Work out the finished part from the listing and answer in its coordinate system (mm). Round coordinates to 2 decimals unless told otherwise and drop trailing zeros. Loops run counter-clockwise (first coordinate to the right, second up) from the corner with the lowest first, then second, coordinate; pieces in that order, holes last. Notation, with made-up numbers: (11.5, 62.5) - (25.5, 62.5) arc R23 ccw to (25.5, 71.5) - close; hole circle Ø9 at (64.5, 83). An arc over 180 degrees is marked (long way). Use CSV: the item, a comma, the result in double quotes. Start each with the question number.
from build123d import *

# Parameters (mm, degrees)
ESQUISSE1_W                                 = 100
ESQUISSE1_H                                 = 100
BOSS_EXTRU_1_DEPTH                          = 1
FRAISAGE_POUR_VIS_T_TE_FRAIS_E_M31_AT_COUNT = 2
FRAISAGE_POUR_VIS_T_TE_FRAIS_E_M31_AT_PITCH = 90
FRAISAGE_POUR_VIS_T_TE_FRAIS_E_M31_2_COUNT  = 2
FRAISAGE_POUR_VIS_T_TE_FRAIS_E_M31_2_PITCH  = 127.279220614
FRAISAGE_POUR_VIS_T_TE_FRAIS_E_M31_3_COUNT  = 2
FRAISAGE_POUR_VIS_T_TE_FRAIS_E_M31_3_PITCH  = 90
ESQUISSE4_R                                 = 5.05
ESQUISSE4_R_2                               = 1
ENL_V_MAT_EXTRU_1_DEPTH                     = 2


with BuildPart() as part:
    # Esquisse1 → Boss.-Extru.1 (new body)
    with BuildSketch(Plane.XY):
        with Locations((50, 50)):
            Rectangle(ESQUISSE1_W, ESQUISSE1_H)
    extrude(amount=BOSS_EXTRU_1_DEPTH)

    # Esquisse3 → Fraisage pour vis à tête fraisée M31 (revolve, cut)
    with BuildSketch(Plane(origin=(5, 95, 1), x_dir=(0, -1, 0), z_dir=(1, 0, 0))):
        Polygon((0, 0), (0, 1), (1.8, 1), (1.8, 1.35), (3.15, 0), align=None)
    fraisage_pour_vis_t_te_frais_e_m31 = revolve(axis=Axis((5, 95, 7.35), (0, 0, -1)), mode=Mode.SUBTRACT)

    # Fraisage pour vis à tête fraisée M31 at: Fraisage pour vis à tête fraisée M31 ×2
    with Locations(*[(i * FRAISAGE_POUR_VIS_T_TE_FRAIS_E_M31_AT_PITCH, 0, 0) for i in range(1, FRAISAGE_POUR_VIS_T_TE_FRAIS_E_M31_AT_COUNT)]):
        add(fraisage_pour_vis_t_te_frais_e_m31, mode=Mode.SUBTRACT)

    # Fraisage pour vis _ t_te frais_e M31 2: Fraisage pour vis à tête fraisée M31 ×2
    with Locations(*[Vector(0.707106781, -0.707106781, 0) * (i * FRAISAGE_POUR_VIS_T_TE_FRAIS_E_M31_2_PITCH) for i in range(1, FRAISAGE_POUR_VIS_T_TE_FRAIS_E_M31_2_COUNT)]):
        add(fraisage_pour_vis_t_te_frais_e_m31, mode=Mode.SUBTRACT)

    # Fraisage pour vis _ t_te frais_e M31 3: Fraisage pour vis à tête fraisée M31 ×2
    with Locations(*[(0, -i * FRAISAGE_POUR_VIS_T_TE_FRAIS_E_M31_3_PITCH, 0) for i in range(1, FRAISAGE_POUR_VIS_T_TE_FRAIS_E_M31_3_COUNT)]):
        add(fraisage_pour_vis_t_te_frais_e_m31, mode=Mode.SUBTRACT)

    # Esquisse4 → Enlèv. mat.-Extru.1 (cut, through all)
    with BuildSketch(Plane.XY.offset(1)):
        with Locations((12.5, 75)):
            Circle(ESQUISSE4_R)
        with Locations((12.5, 25)):
            Circle(ESQUISSE4_R_2)
        with Locations((10, 19.5)):
            Circle(ESQUISSE4_R_2)
        with Locations((7, 25)):
            Circle(ESQUISSE4_R_2)
        with Locations((18, 25)):
            Circle(ESQUISSE4_R_2)
        with Locations((10, 30.5)):
            Circle(ESQUISSE4_R_2)
        with Locations((15, 30.5)):
            Circle(ESQUISSE4_R_2)
        with Locations((15, 19.5)):
            Circle(ESQUISSE4_R_2)
        with Locations((12.5, 60)):
            Circle(ESQUISSE4_R)
        with Locations((12.5, 45)):
            Circle(ESQUISSE4_R)
    extrude(amount=-ENL_V_MAT_EXTRU_1_DEPTH, mode=Mode.SUBTRACT)


solid = part.part
Item 1: A cutting plane is placed at D-D (y = 43). Determine the outline of the cut face in (x, z).
Item 2: A cutting plane is placed at C-C (y = 60). Determine the outline of the cut face in (x, z).
Item 3: A cutting plane is placed at B-B (z = 0.7). State how many separate pieces and enclosed holes the cut face has, plus the area to 3 significant figures.
Item 4: A cutting plane is placed at A-A (y = 5). Determine the outline of the cut face in (x, z).
Item 5: Find the intervals of material crossed by probe 1 along Y at (x, z) = (12.5, 0.4); probe 2 along Y at (x, z) = (15, 0.65); probe 3 along X at (y, z) = (49, 0.8), in increasing order. Write a range as [from, to].
Item 6: The mould has two halves that part along Y. Classify faces 1 (the cylindrical face through (14.83, 55.52, 0.51)), 2 (the flat face through (49, 51, 1)): pulls with the +Y half, pulls with the -Y half, needs draft (parallel to the pull), parting line crosses it, or undercut.
Result sheet:
1,outline,"(0, 0) - (7.86, 0) - (7.86, 1) - (0, 1) - close; (17.14, 0) - (100, 0) - (100, 1) - (17.14, 1) - close"
2,outline,"(0, 0) - (7.45, 0) - (7.45, 1) - (0, 1) - close; (17.55, 0) - (100, 0) - (100, 1) - (17.55, 1) - close"
3,separate pieces,"1"
3,enclosed holes,"14"
3,area,"9,640 mm^2"
4,outline,"(0, 0) - (2.85, 0) - (1.85, 1) - (0, 1) - close; (7.15, 0) - (92.85, 0) - (91.85, 1) - (8.15, 1) - close; (97.15, 0) - (100, 0) - (100, 1) - (98.15, 1) - close"
5,probe 1,"[0, 24], [26, 39.95], [50.05, 54.95], [65.05, 69.95], [80.05, 100]"
5,probe 2,"[0, 18.5], [20.5, 29.5], [31.5, 40.61], [49.39, 55.61], [64.39, 70.61], [79.39, 100]"
5,probe 3,"[0, 9.42], [15.58, 100]"
6,face 1,"undercut"
6,face 2,"needs draft"
